Could you check a few things on this model? Use its own coordinates, in mm. Give positions to 0.01 mm unless a question says otherwise; leave off trailing zeros. Write each loop counter-clockwise with the first axis right and the second up, starting at its lowest first coordinate (ties: lowest second). Pieces come first, ordered by that corner, then holes. Notation, with made-up numbers: (17, 17.25) - (74, 17.25) arc R21 ccw to (74, 44.25) - close; hole circle Ø7 at (-4, 22.25). An arc over 180 degrees is marked (long way). Answer in a Markdown table with one row per item.
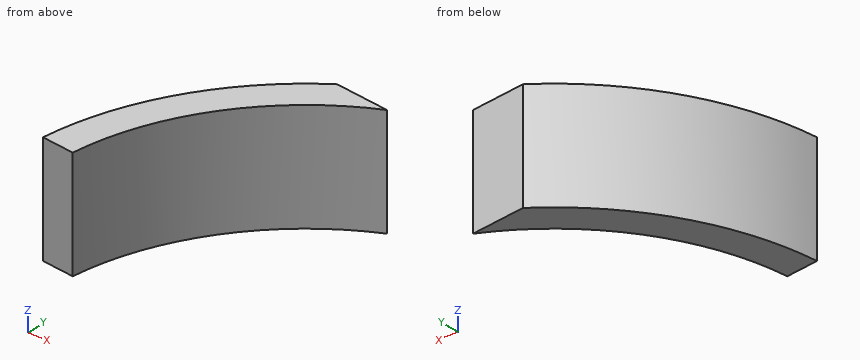
from build123d import *

# Parameters (mm, degrees)
EXTRUDE_1_DEPTH          = 6.15
CUT_EXTRUDE_1_DEPTH      = 17.072414255
CUT_EXTRUDE_1_DEPTH_BACK = 17.072414255


with BuildPart() as part:
    # 草图1 → 凸台-拉伸1 (new body)
    with BuildSketch(Plane.XY):
        with BuildLine():
            Line((-9.3, 0), (-10.5, 0))
            ThreePointArc((-10.5, 0), (-0.549527541, 10.485610115), (10.442479901, 1.097548864))
            Line((10.442479901, 1.097548864), (9.249053627, 0.972114708))
            ThreePointArc((9.249053627, 0.972114708), (-0.486724393, 9.287254673), (-9.3, 0))
        make_face()
    extrude(amount=EXTRUDE_1_DEPTH)

    # 草图4 → 切除-拉伸1 (cut, two sides)
    with BuildSketch(Plane(origin=(0, 0, 6.15), x_dir=(0, 0, 1), z_dir=(-0.9945218953682734, 0.10452846326765432, 0))) as cut_extrude_1_sk:
        Polygon((0, -0.097548864), (-4, -0.097548864), (-4, 7.902451136), (0, 7.902451136), (0, 10.5), (-6.15, 10.5), (-6.15, -1.097548864), (0, -1.097548864), align=None)
    extrude(amount=CUT_EXTRUDE_1_DEPTH, mode=Mode.SUBTRACT)
    extrude(cut_extrude_1_sk.sketch, amount=-CUT_EXTRUDE_1_DEPTH_BACK, mode=Mode.SUBTRACT)


with BuildPart() as body_2:
    # of the pieces the cut leaves, the one that is kept (cut_extrude_1_keep)
    add(part.part.solids().sort_by_distance((-4.050298117, 8.371683532, 6.15))[0])


solid = body_2.part
1) If I drill on line 1 (X direction, y = 7, z = 5.1); line 2 (Y direction, x = -5, z = 3.75); line 3 (Y direction, x = -5.5, z = 4.75), over which ranges is the centre line in solid material (lowest first)?
Check values:
| item | result |
|---|---|
| line 1 | x = -7.83 to -6.12 |
| line 2 | y = 7.84 to 8.47 |
| line 3 | y = 7.5 to 8.52 |
2) Imagine slicing it at A-A (z = 5.95). List the corners of the cut face in (x, y) for me.
Check values:
| item | result |
|---|---|
| outline | (-10.45, 1) - (-9.26, 0.88) arc R9.3 cw to (-4.05, 8.37) - (-6.05, 8.58) arc R10.5 ccw to start |
3) Imagine slicing it at B-B (x = -8.5). List the corners of the cut face in (y, z) for me.
Check values:
| item | result |
|---|---|
| outline | (3.77, 2.15) - (6.16, 2.15) - (6.16, 6.15) - (3.77, 6.15) - close |
4) Will these pins go through, and if not, where does the flat tip stop? P1, Ø1.5, axis at y = 2, z = 5.5, coming from the +X side; P2, Ø1.5, axis at y = 5, z = 3, coming from the +X side.
Check values:
| item | result |
|---|---|
| P1 | stops at x = -8.88 |
| P2 | stops at x = -7.31 |
